Check sheet for the modelled part. Datum: model origin and axes. Units: mm. A direction names the side the tool comes from. Round coordinates to 2 decimals unless told otherwise and drop trailing zeros. Loops run counter-clockwise (first coordinate to the right, second up) from the corner with the lowest first, then second, coordinate; pieces in that order, holes last. Notation, with made-up numbers: (55, 82) -> (71, 82) arc R25 cw to (71, 112) -> close; hole circle Ø3 at (45.25, 34.5). An arc over 180 degrees is marked (long way). One line per item, written item: value. Start each with the question number.
1. Set-up check for faces 1 (the face through (60, -5, 51)), 2 (the face through (-1, 2, 48)), 3 (the face through (66, 0, -1)): record each of +Z, -Z, +X, -X, +Y, -Y from which the full face is reachable in a straight line by a thin tool's end or side.
2. Material ranges on L1, parallel to X at y = 1.75, z = 1.5; L2, parallel to Z at x = 45.5, y = 0.75; L3, parallel to Y at x = 5.5, z = -52.5, recorded low to high.
3. Cross-section at B-B on y = -3.5. Record the cut outline in (x, z), then the cut area to 3 significant figures.
4. Go/stop test with flat-tipped pins: pin 1 (1 mm diameter, centred on x = -7, y = -1.5, fed in from -Z); pin 2 (14.5 mm diameter, centred on x = 65, z = -16.5, fed in from -Y). Record where each tip stops, or that it passes through.
5. Release check for a two-part mould opening along Z. For faces 4 (the face through (-60, -5, -52)), 5 (the face through (66, -5, 45)), 6 (the face through (-1, 1, -58)), 7 (the face through (-1, 1, 58)) record: +Z half, -Z half, draft (parallel to the pull), parting line (faces both ways), or undercut.
6. Cross-section at A-A on x = 51. Record the cut outline in (y, z), then the cut area to 3 significant figures.
7. Cross-section at C-C on z = -25. Record the cut outline in (x, y), then the cut area to 3 significant figures.
from build123d import *

# Parameters (mm, degrees)
SKETCH1_W      = 146
SKETCH1_H      = 116
SKETCH1_W_2    = 140
SKETCH1_H_2    = 110
DINDING_DEPTH  = 3
SKETCH1_4_W    = 140
SKETCH1_4_H    = 110
SKETCH1_4_W_2  = 120
SKETCH1_4_H_2  = 90
LANDSITE_DEPTH = 2
SKETCH2_W      = 13
SKETCH2_H      = 13
KAKI_DEPTH     = 10


with BuildPart() as part:
    # Sketch1 → Dinding (new body)
    with BuildSketch(Plane(origin=(0, 0, 0), x_dir=(1, 0, 0), z_dir=(0, 1, 0))):
        Rectangle(SKETCH1_W, SKETCH1_H)
        Rectangle(SKETCH1_W_2, SKETCH1_H_2, mode=Mode.SUBTRACT)
    extrude(amount=DINDING_DEPTH)

    # Sketch1<4> → Landsite (add)
    with BuildSketch(Plane(origin=(0, 0, 0), x_dir=(1, 0, 0), z_dir=(0, 1, 0))):
        Rectangle(SKETCH1_4_W, SKETCH1_4_H)
        Rectangle(SKETCH1_4_W_2, SKETCH1_4_H_2, mode=Mode.SUBTRACT)
    extrude(amount=LANDSITE_DEPTH)

    # Sketch2 → Kaki (add)
    with BuildSketch(Plane.XZ):
        with Locations((-66.5, 51.5)):
            Rectangle(SKETCH2_W, SKETCH2_H)
        with Locations((-66.5, -51.5)):
            Rectangle(SKETCH2_W, SKETCH2_H)
        with Locations((66.5, -51.5)):
            Rectangle(SKETCH2_W, SKETCH2_H)
        with Locations((66.5, 51.5)):
            Rectangle(SKETCH2_W, SKETCH2_H)
    extrude(amount=KAKI_DEPTH)


solid = part.part
Taken from the geometry:
1. face 1: +Z, -Z, -Y
1. face 2: +Y
1. face 3: +X, -X, -Y
2. L1: x = -73 to -60, 60 to 73
2. L2: z = -58 to -45, 45 to 58
2. L3: y = 0 to 2
3. outline: (-73, -58) -> (-60, -58) -> (-60, -45) -> (-73, -45) -> close; (-73, 45) -> (-60, 45) -> (-60, 58) -> (-73, 58) -> close; (60, -58) -> (73, -58) -> (73, -45) -> (60, -45) -> close; (60, 45) -> (73, 45) -> (73, 58) -> (60, 58) -> close
3. area: 676 mm2
4. pin 1: passes through
4. pin 2: stops at y = 0
5. face 4: draft
5. face 5: undercut
5. face 6: -Z half
5. face 7: +Z half
6. outline: (0, -58) -> (3, -58) -> (3, -55) -> (2, -55) -> (2, -45) -> (0, -45) -> close; (0, 45) -> (2, 45) -> (2, 55) -> (3, 55) -> (3, 58) -> (0, 58) -> close
6. area: 58.0 mm2
7. outline: (-73, 0) -> (-60, 0) -> (-60, 2) -> (-70, 2) -> (-70, 3) -> (-73, 3) -> close; (60, 0) -> (73, 0) -> (73, 3) -> (70, 3) -> (70, 2) -> (60, 2) -> close
7. area: 58.0 mm2
